```python
from build123d import *

# Parameters (mm, degrees)
F1_DEPTH = 25.4


with BuildPart() as f1:
    # F0 (on Right) → F1 (new body)
    with BuildSketch(Plane.YZ):
        with BuildLine():
            Line((-22.8805579245, -22.7664159755), (-22.8805579245, -57.9928606749))
            Line((-22.8805579245, -57.9928606749), (-15.3976082802, -57.9928606749))
            Line((-15.3976082802, -57.9928606749), (-15.3976082802, -30.0726670171))
            ThreePointArc((-15.3976082802, -30.0726670171), (-19.2448601213, -26.5278766879), (-22.8805579245, -22.7664159755))
        make_face()
        with BuildLine():
            ThreePointArc((-36.1290082754, -3.8675027801), (-30.1105807858, -13.7416335631), (-22.8805579245, -22.7664159755))
            Line((-22.8805579245, -22.7664159755), (-22.8805579245, -5.4353086614))
            ThreePointArc((-22.8805579245, -5.4353086614), (-25.2060971884, -1.990536454), (-25.8564343771, 2.1145396683))
            ThreePointArc((-25.8564343771, 2.1145396683), (-30.6840356791, -1.4065674169), (-36.1290082754, -3.8675027801))
        make_face()
        with BuildLine():
            ThreePointArc((-45.277106552, 52.8451455313), (-74.0603906155, 19.1080787818), (-36.1290082754, -3.8675027801))
            ThreePointArc((-36.1290082754, -3.8675027801), (-40.2966096051, 5.2739283062), (-43.4237891642, 14.8214626034))
            ThreePointArc((-43.4237891642, 14.8214626034), (-48.9964160146, 26.897956874), (-46.4641223034, 39.9548850136))
            ThreePointArc((-46.4641223034, 39.9548850136), (-46.1017075688, 46.4212957732), (-45.277106552, 52.8451455313))
        make_face()
        with BuildLine():
            Line((-22.8805579245, -5.4353086614), (-22.8805579245, -22.7664159755))
            ThreePointArc((-22.8805579245, -22.7664159755), (-19.2448601213, -26.5278766879), (-15.3976082802, -30.0726670171))
            Line((-15.3976082802, -30.0726670171), (-15.3976082802, -8.0253607773))
            ThreePointArc((-15.3976082802, -8.0253607773), (-19.4187756139, -7.5383976022), (-22.8805579245, -5.4353086614))
        make_face()
        with BuildLine():
            ThreePointArc((-37.6985580456, 51.8270156729), (-41.4542478809, 52.5860694794), (-45.277106552, 52.8451455313))
            ThreePointArc((-45.277106552, 52.8451455313), (-46.1017075688, 46.4212957732), (-46.4641223034, 39.9548850136))
            ThreePointArc((-46.4641223034, 39.9548850136), (-43.4730918643, 44.1250016569), (-39.5852366825, 47.474735675))
            ThreePointArc((-39.5852366825, 47.474735675), (-38.7160866571, 49.6830361403), (-37.6985580456, 51.8270156729))
        make_face()
        with BuildLine():
            ThreePointArc((-43.4237891642, 14.8214626034), (-40.2966096051, 5.2739283062), (-36.1290082754, -3.8675027801))
            ThreePointArc((-36.1290082754, -3.8675027801), (-30.6840356791, -1.4065674169), (-25.8564343771, 2.1145396683))
            ThreePointArc((-25.8564343771, 2.1145396683), (-25.5163637625, 4.1239695154), (-24.7595102264, 6.0162245347))
            ThreePointArc((-24.7595102264, 6.0162245347), (-26.1371840828, 6.8924645223), (-27.4722746733, 7.8323128533))
            ThreePointArc((-27.4722746733, 7.8323128533), (-36.1811250997, 9.6537304893), (-43.4237891642, 14.8214626034))
        make_face()
        with BuildLine():
            Line((-15.3976082802, -8.0253607773), (-15.3976082802, -30.0726670171))
            ThreePointArc((-15.3976082802, -30.0726670171), (81.3685508669, -44.1009938677), (134.2632217545, 38.1342619658))
            ThreePointArc((134.2632217545, 38.1342619658), (51.2704704846, 128.2052611604), (-45.277106552, 52.8451455313))
            ThreePointArc((-45.277106552, 52.8451455313), (-41.4542478809, 52.5860694794), (-37.6985580456, 51.8270156729))
            ThreePointArc((-37.6985580456, 51.8270156729), (-0.4432478699, 70.0792033475), (27.8432110431, 39.7316048698))
            ThreePointArc((27.8432110431, 39.7316048698), (56.2702105218, 30.9904843235), (68.5100917864, 3.8853778969))
            ThreePointArc((68.5100917864, 3.8853778969), (39.6372370921, -31.5098645214), (-0.8370252167, -10.336791655))
            ThreePointArc((-0.8370252167, -10.336791655), (-6.0781786291, -9.3223624176), (-10.0928384047, -5.8036605751))
            ThreePointArc((-10.0928384047, -5.8036605751), (-12.5748209934, -7.3213816154), (-15.3976082802, -8.0253607773))
        make_face()
        with BuildLine():
            ThreePointArc((1.9137445003, -9.7472674078), (0.558740927, -10.1371303225), (-0.8370252167, -10.336791655))
            ThreePointArc((-0.8370252167, -10.336791655), (39.6372370921, -31.5098645214), (68.5100917864, 3.8853778969))
            ThreePointArc((68.5100917864, 3.8853778969), (56.2702105218, 30.9904843235), (27.8432110431, 39.7316048698))
            ThreePointArc((27.8432110431, 39.7316048698), (28.0074467559, 37.7847839297), (28.0622494863, 35.8318164945))
            ThreePointArc((28.0622494863, 35.8318164945), (26.1412305096, 24.4251830851), (20.5901041712, 14.2769519082))
            ThreePointArc((20.5901041712, 14.2769519082), (20.6380886941, 13.9210160561), (20.6769120054, 13.5639648052))
            ThreePointArc((20.6769120054, 13.5639648052), (20.8650675932, 13.24447129), (21.0457330933, 12.9206833832))
            ThreePointArc((21.0457330933, 12.9206833832), (28.9159774204, 10.9365568541), (32.3825042542, 3.597572213))
            ThreePointArc((32.3825042542, 3.597572213), (28.0844870819, -4.352654537), (19.0786813985, -5.1106261617))
            ThreePointArc((19.0786813985, -5.1106261617), (11.203643005, -10.0478667355), (1.9137445003, -9.7472674078))
        make_face()
    extrude(amount=F1_DEPTH)


solid = f1.part
```
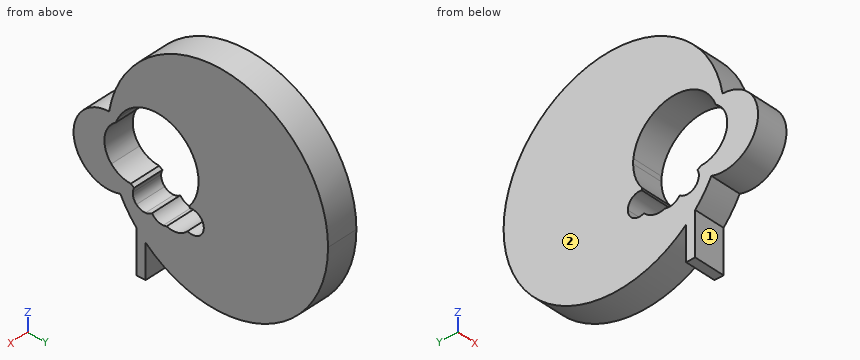
Geometry: final body of the model. Coordinates: model frame, mm. Face numbers are marked on the shaded views. A direction names the side the tool comes from. Coordinates: 2 decimals unless noted, no trailing zeros. Write each loop counter-clockwise with the first axis right and the second up, starting at its lowest first coordinate (ties: lowest second). Pieces come first, ordered by that corner, then holes. Notation, with made-up numbers: M 9.5,-1.75 L 34.5,-1.75 A29 cw 34.5,36.25 Z; hole C 37.5,-35.75 d2. An arc over 180 degrees is marked long. Use CSV: the item, a comma, the result in double quotes. Start each with the question number.
1. Cut plane B-B on x = 18. Return the cut outline in (y, z), plus the area to 3 significant figures.
2. Ray query, probe 1 along Z at (x, y) = (22.75, -23); probe 2 along Z at (x, y) = (12.5, -7.5); probe 3 along Y at (x, z) = (2.25, -41.5). Return the intervals inside material, ascending.
3. Cut plane A-A on z = 45. Return the cut outline in (x, y), plus the area to 3 significant figures.
4. Cut plane D-D on y = 62. Return the cut outline in (x, z), plus the area to 3 significant figures.
5. Cut plane C-C on z = 20. Return the cut outline in (x, y), plus the area to 3 significant figures.
6. Reachability of the marked faces 1 and 2 from +Z, -Z, +X, -X, +Y, -Y: full face, straight path, thin tool, end or side. Return the list, or none.
7. First-contact query: P1, Ø2, axis at x = 3.5, z = 85.5, coming from the -Y side; P2, Ø8, axis at x = 7, y = -6.5, coming from the -Z side; P3, Ø10, axis at x = 4.5, z = 57.5, coming from the +Y side. Flat tips, straight axial feed; report the tip coordinate or a pass-through.
Entries:
1,outline,"M -45.28,52.85 A29.1 ccw long -36.13,-3.87 A90.37 ccw -22.88,-22.77 L -22.88,-57.99 L -15.4,-57.99 L -15.4,-30.07 A90.37 ccw long Z; hole M -39.59,47.47 A21.67 ccw -27.47,7.83 A34.83 ccw -24.76,6.02 A9.59 ccw -10.09,-5.8 A10.22 ccw 1.91,-9.75 A15.92 ccw 19.08,-5.11 A9.5 ccw long 21.05,12.92 A15.92 ccw 20.68,13.56 A13.98 ccw 20.59,14.28 A34.83 ccw long Z"
1,area,"22,500 mm²"
2,probe 1,"-22.64 to -5.32, 66.64 to 98.9"
2,probe 2,"-36.2 to -8.48, 70.65 to 112.47"
2,probe 3,"-22.88 to -15.4, 1.16 to 86.62"
3,outline,"M 0,-65.21 L 25.4,-65.21 L 25.4,-42.63 L 0,-42.63 Z; M 0,26.83 L 25.4,26.83 L 25.4,134 L 0,134 Z"
3,area,"3,300 mm²"
4,outline,"M 0,-50.41 L 25.4,-50.41 L 25.4,126.67 L 0,126.67 Z"
4,area,"4,500 mm²"
5,outline,"M 0,-74.19 L 25.4,-74.19 L 25.4,-46.96 L 0,-46.96 Z; M 0,24.26 L 25.4,24.26 L 25.4,132.43 L 0,132.43 Z"
5,area,"3,440 mm²"
6,face 1,"-Z, +X, -X, -Y"
6,face 2,"+Z, -Z, -X, +Y, -Y"
7,P1,"y = -33.68"
7,P2,"z = -39.42"
7,P3,"y = 133.11"
